Verification items for the finished model (mm, model axes). A direction names the side the tool comes from. Give positions to 0.01 mm unless a question says otherwise; leave off trailing zeros. Order: outer loops, then holes, each group sorted by start corner. A loop starts at its lowest first (then second) coordinate and runs counter-clockwise, first axis right, second up. Notation, with made-up numbers: M 21,31 L 77,31 A29 ccw 77,68 Z; hole C -9.75,-11 d10. An arc over 180 degrees is marked long. Answer as a JSON object with one key per item and string values.
```python
from build123d import *

# Parameters (mm, degrees)
SKETCH4_W           = 60
SKETCH4_H           = 14
BOSS_EXTRUDE2_DEPTH = 3
BOSS_EXTRUDE3_REACH = 63.685
SKETCH7_W           = 4
SKETCH7_H           = 10
CUT_EXTRUDE2_DEPTH  = 63.128898268
SKETCH8_R           = 1.75
CUT_EXTRUDE3_DEPTH  = 63.265560304
CUT_EXTRUDE4_START  = -1
SKETCH9_R           = 3
CUT_EXTRUDE4_DEPTH  = 1.5
FILLET1_R           = 1.5


with BuildPart() as part:
    # Sketch4 → Boss-Extrude2 (new body)
    with BuildSketch(Plane.YZ):
        with Locations((30, 7)):
            Rectangle(SKETCH4_W, SKETCH4_H)
        with BuildLine():
            Line((6.5, 9.5), (53.5, 9.5))
            ThreePointArc((53.5, 9.5), (56, 7), (53.5, 4.5))
            Line((53.5, 4.5), (6.5, 4.5))
            ThreePointArc((6.5, 4.5), (4, 7), (6.5, 9.5))
        make_face(mode=Mode.SUBTRACT)
    extrude(amount=BOSS_EXTRUDE2_DEPTH)

    # Boss-Extrude3: up to this face of the body (flat: up to its plane)
    boss_extrude3_end = Plane(part.part.faces().sort_by_distance((1.5, 30, 14))[0])
    # Sketch6 → Boss-Extrude3 (add, up to the picked face)
    with BuildSketch(Plane(origin=(0, 0, 0), x_dir=(1, 0, 0), z_dir=(0, 0, -1)), mode=Mode.PRIVATE) as boss_extrude3_sk1:
        Polygon((0, -2.828427125), (-6, -8.828427125), (-6, -13.828427125), (0, -19.828427125), (0, -22.656854249), (-8, -14.656854249), (-8, -8), (0, 0), align=None)
    boss_extrude3_tool1 = split(extrude(boss_extrude3_sk1.sketch, amount=-BOSS_EXTRUDE3_REACH, mode=Mode.PRIVATE), bisect_by=boss_extrude3_end, keep=Keep.BOTH, mode=Mode.PRIVATE)
    # Sketch6 → Boss-Extrude3 (add, up to the picked face)
    with BuildSketch(Plane(origin=(0, 0, 0), x_dir=(1, 0, 0), z_dir=(0, 0, -1)), mode=Mode.PRIVATE) as boss_extrude3_sk2:
        Polygon((0, -33.828427125), (-6, -39.828427125), (-6, -44.828427125), (0, -50.828427125), (0, -53.656854249), (-8, -45.656854249), (-8, -39), (0, -31), align=None)
    boss_extrude3_tool2 = split(extrude(boss_extrude3_sk2.sketch, amount=-BOSS_EXTRUDE3_REACH, mode=Mode.PRIVATE), bisect_by=boss_extrude3_end, keep=Keep.BOTH, mode=Mode.PRIVATE)
    add(boss_extrude3_tool1.solids().sort_by(Axis((-3.169902, 5.658525, 0), (0, 0, 1)))[0])
    add(boss_extrude3_tool2.solids().sort_by(Axis((-3.169902, 36.658525, 0), (0, 0, 1)))[0])

    # Sketch7 → Cut-Extrude2 (cut, through all)
    with BuildSketch(Plane(origin=(0, 60, 0), x_dir=(-1, 0, 0), z_dir=(0, 1, 0))):
        with Locations((2, 7)):
            Rectangle(SKETCH7_W, SKETCH7_H)
    extrude(amount=-CUT_EXTRUDE2_DEPTH, mode=Mode.SUBTRACT)

    # Sketch8 → Cut-Extrude3 (cut, through all)
    with BuildSketch(Plane.YZ.offset(-6)):
        with Locations((42.328427125, 7)):
            Circle(SKETCH8_R)
        with Locations((11.328427125, 7)):
            Circle(SKETCH8_R)
    extrude(amount=-CUT_EXTRUDE3_DEPTH, mode=Mode.SUBTRACT)

    # Sketch9 → Cut-Extrude4 (cut)
    with BuildSketch(Plane.YZ.offset(-6).offset(CUT_EXTRUDE4_START)):
        with Locations(Location((11.328427125, 7, 0), (0, 0, 270))):
            Circle(SKETCH9_R)
        with Locations(Location((42.328427125, 7, 0), (0, 0, 213.557309762))):
            Circle(SKETCH9_R)
    extrude(amount=CUT_EXTRUDE4_DEPTH, mode=Mode.SUBTRACT)

    # Fillet1
    fillet1_edges = [part.edges().sort_by_distance(p)[0] for p in [
        (0, 53.656854249, 1),
        (0, 53.656854249, 13),
        (0, 33.828427125, 13),
        (0, 50.828427125, 13),
        (0, 31, 13),
        (0, 50.828427125, 1),
        (0, 33.828427125, 1),
        (0, 2.828427125, 13),
        (0, 19.828427125, 13),
        (0, 19.828427125, 1),
        (0, 2.828427125, 1),
        (-6, 13.828427125, 11.329156198),
        (-6, 8.828427125, 11.329156198),
        (-6, 8.828427125, 2.670843802),
        (-6, 13.828427125, 2.670843802),
    ]]
    fillet(fillet1_edges, radius=FILLET1_R)


solid = part.part
```
Q1. Material ranges on L1, parallel to Y at x = -6.45, z = 7; L2, parallel to X at y = 13, z = 9.75; L3, parallel to Y at x = -6.5, z = 7, recorded low to high.
Resolved:
{"L1": "y = 6.45 to 8.33, 14.33 to 16.21, 37.45 to 39.33, 45.33 to 47.21", "L2": "x = -8 to -6, 0 to 3", "L3": "y = 6.5 to 8.33, 14.33 to 16.16, 37.5 to 39.33, 45.33 to 47.16"}
Q2. Section check B-B on z = 3. Record the cut outline in (x, y), then the cut area to 3 significant figures.
Resolved:
{"outline": "M -8,8 L -4,4 L -4,6.83 L -5.56,8.39 A1.5 cw -6,9.45 L -6,13.21 A1.5 cw -5.56,14.27 L -4,15.83 L -4,18.66 L -8,14.66 Z; M -8,39 L -4,35 L -4,37.83 L -6,39.83 L -6,44.83 L -4,46.83 L -4,49.66 L -8,45.66 Z; M 0,0 L 3,0 L 3,60 L 0,60 Z", "area": "237 mm²"}
Q3. Release check for a two-part mould opening along X. For faces 1 (the face through (1, 60, 7)), 2 (the face through (-8, 11, 5)), 3 (the face through (-4.415, 15.413, 6.902)) record: +X half, -X half, draft (parallel to the pull), parting line (faces both ways), or undercut.
Resolved:
{"face 1": "draft", "face 2": "-X half", "face 3": "undercut"}
Q4. Tool access check on faces 4 (the face through (-0.949, 36.055, 13.014)), 5 (the face through (-7.493, 12.945, 6.33)), 6 (the face through (0, 30, 4)), 7 (the face through (-4, 36, 7)). Record the directions out of +Z, -Z, +X, -X, +Y, -Y that give a thin tool (end or side, any length) a straight path to the whole face; none if there is none.
Resolved:
{"face 4": "+Z, -Z", "face 5": "+X, -X", "face 6": "none", "face 7": "+Y, -Y"}
Q5. Section check A-A on x = 1. Record the cut outline in (y, z), then the cut area to 3 significant figures.
Resolved:
{"outline": "M 0,0 L 60,0 L 60,14 L 0,14 Z; hole M 6.5,4.5 L 53.5,4.5 A2.5 ccw 53.5,9.5 L 6.5,9.5 A2.5 ccw Z", "area": "585 mm²"}
